from build123d import *

# Parameters (mm, degrees)
SKETCH1_R           = 10
SKETCH1_R_2         = 7.25
BOSS_EXTRUDE2_DEPTH = 10
SKETCH2_R           = 7.25
CUT_EXTRUDE1_DEPTH  = 10
CHAMFER5_SIZE       = 2.5
SKETCH5_W           = 6.2
SKETCH5_H           = 2
BOSS_EXTRUDE3_DEPTH = 8.5
SKETCH6_W           = 2.931408159
SKETCH6_H           = 6.9
BOSS_EXTRUDE4_DEPTH = 10
SKETCH7_W           = 8.5
SKETCH7_H           = 6.2
CUT_EXTRUDE2_DEPTH  = 1
SKETCH8_R           = 1.35
CUT_EXTRUDE3_DEPTH  = 20
BOSS_EXTRUDE5_START = -10
BOSS_EXTRUDE5_DEPTH = 10
SKETCH12_W          = 20
SKETCH12_H          = 10
SKETCH12_W_2        = 18
SKETCH12_H_2        = 8
BOSS_EXTRUDE7_DEPTH = 12
SKETCH13_W          = 10.931408159
SKETCH13_H          = 4.9
CUT_EXTRUDE4_DEPTH  = 9
SKETCH15_W          = 20
SKETCH15_H          = 10
SKETCH15_W_2        = 18
SKETCH15_H_2        = 8
CUT_EXTRUDE5_DEPTH  = 5


with BuildPart() as part:
    # Sketch1 → Boss-Extrude2 (new body)
    # profile 1 of 3: a face of its own
    with BuildSketch(Plane(origin=(0, 0, 0), x_dir=(1, 0, 0), z_dir=(0, 1, 0))):
        with Locations((-21.149759624, -29.701544489)):
            Circle(SKETCH1_R)
        with Locations((-21.149759624, -29.701544489)):
            Circle(SKETCH1_R_2, mode=Mode.SUBTRACT)
    # profile 2 of 3: a face of its own
    with BuildSketch(Plane(origin=(0, 0, 0), x_dir=(1, 0, 0), z_dir=(0, 1, 0))):
        with Locations((-21.149759624, -29.701544489)):
            Circle(SKETCH1_R_2)
    # profile 3 of 3: a face of its own
    with BuildSketch(Plane(origin=(0, 0, 0), x_dir=(1, 0, 0), z_dir=(0, 1, 0))):
        with BuildLine():
            Line((-1.149759624, -19.701544489), (-21.149759624, -19.701544489))
            ThreePointArc((-21.149759624, -19.701544489), (-14.078691812, -22.630476677), (-11.149759624, -29.701544489))
            ThreePointArc((-11.149759624, -29.701544489), (-14.078691797, -36.772612285), (-21.149759581, -39.701544489))
            Line((-21.149759581, -39.701544489), (-1.149759624, -39.701544489))
            Line((-1.149759624, -39.701544489), (-1.149759624, -32.801544489))
            Line((-1.149759624, -32.801544489), (-6.718351465, -32.801544489))
            Line((-6.718351465, -32.801544489), (-6.718351465, -26.601544489))
            Line((-6.718351465, -26.601544489), (-1.149759624, -26.601544489))
            Line((-1.149759624, -26.601544489), (-1.149759624, -19.701544489))
        make_face()
    extrude(amount=BOSS_EXTRUDE2_DEPTH)

    # Sketch2 → Cut-Extrude1 (cut)
    with BuildSketch(Plane(origin=(0, 10, 0), x_dir=(1, 0, 0), z_dir=(0, 1, 0))):
        with Locations(Location((-21.149759624, -29.701544489, 0), (0, 0, 270))):
            Circle(SKETCH2_R)
    extrude(amount=-CUT_EXTRUDE1_DEPTH, mode=Mode.SUBTRACT)

    # Chamfer5
    chamfer5_edges = [part.edges().sort_by_distance(p)[0] for p in [
        (-21.149759624, 0, 22.451544489),
        (-21.149759624, 10, 22.451544489),
    ]]
    chamfer(chamfer5_edges, length=CHAMFER5_SIZE)

    # Sketch5 → Boss-Extrude3 (add)
    with BuildSketch(Plane(origin=(-6.718351465, 0, 0), x_dir=(0, 0, -1), z_dir=(1, 0, 0))):
        with Locations((-29.701544489, 9)):
            Rectangle(SKETCH5_W, SKETCH5_H)
    extrude(amount=BOSS_EXTRUDE3_DEPTH)

    # Sketch6 → Boss-Extrude4 (add)
    with BuildSketch(Plane(origin=(0, 10, 0), x_dir=(1, 0, 0), z_dir=(0, 1, 0))):
        with Locations((0.315944456, -23.151544489)):
            Rectangle(SKETCH6_W, SKETCH6_H)
        with Locations((0.315944456, -36.251544489)):
            Rectangle(SKETCH6_W, SKETCH6_H)
    extrude(amount=-BOSS_EXTRUDE4_DEPTH)

    # Sketch7 → Cut-Extrude2 (cut)
    with BuildSketch(Plane.XZ.offset(-8)):
        with Locations((-2.468351465, 29.701544489)):
            Rectangle(SKETCH7_W, SKETCH7_H)
    extrude(amount=-CUT_EXTRUDE2_DEPTH, mode=Mode.SUBTRACT)

    # Sketch8 → Cut-Extrude3 (cut)
    with BuildSketch(Plane.XY.offset(39.701544489)):
        with Locations((-2.868351465, 5)):
            Circle(SKETCH8_R)
    extrude(amount=-CUT_EXTRUDE3_DEPTH, mode=Mode.SUBTRACT)

    # Sketch10 → Boss-Extrude5 (add)
    with BuildSketch(Plane(origin=(0, 10, 0), x_dir=(1, 0, 0), z_dir=(0, 1, 0)).offset(BOSS_EXTRUDE5_START)):
        with BuildLine():
            ThreePointArc((-31.149759624, -29.701544489), (-28.220827436, -22.630476677), (-21.149759624, -19.701544489))
            Line((-21.149759624, -19.701544489), (-31.149759624, -19.701544489))
            Line((-31.149759624, -19.701544489), (-31.149759624, -29.701544489))
        make_face()
        with BuildLine():
            ThreePointArc((-21.149759624, -39.701544489), (-28.220827436, -36.772612301), (-31.149759624, -29.701544489))
            Line((-31.149759624, -29.701544489), (-31.149759624, -39.701544489))
            Line((-31.149759624, -39.701544489), (-21.149759624, -39.701544489))
        make_face()
    extrude(amount=BOSS_EXTRUDE5_DEPTH)

    # Sketch12 → Boss-Extrude7 (add)
    with BuildSketch(Plane.ZY.offset(31.149759624)):
        with Locations((29.701544489, 5)):
            Rectangle(SKETCH12_W, SKETCH12_H)
        with Locations((29.701544489, 5)):
            Rectangle(SKETCH12_W_2, SKETCH12_H_2, mode=Mode.SUBTRACT)
    extrude(amount=BOSS_EXTRUDE7_DEPTH)

    # Sketch13 → Cut-Extrude4 (cut)
    with BuildSketch(Plane.XZ):
        with Locations((-4.684055545, 23.151544489)):
            Rectangle(SKETCH13_W, SKETCH13_H)
        Polygon((-13.850581564, 20.701544489), (-10.149759624, 25.601544489), (-10.149759624, 20.701544489), align=None)
        with Locations((-4.684055545, 36.251544489)):
            Rectangle(SKETCH13_W, SKETCH13_H)
        Polygon((-13.850581564, 38.701544489), (-10.149759624, 38.701544489), (-10.149759624, 33.801544489), align=None)
    extrude(amount=-CUT_EXTRUDE4_DEPTH, mode=Mode.SUBTRACT)

    # Sketch15 → Cut-Extrude5 (cut)
    with BuildSketch(Plane.ZY.offset(43.149759624)):
        with Locations((29.701544489, 5)):
            Rectangle(SKETCH15_W, SKETCH15_H)
        with Locations((29.701544489, 5)):
            Rectangle(SKETCH15_W_2, SKETCH15_H_2, mode=Mode.SUBTRACT)
    extrude(amount=-CUT_EXTRUDE5_DEPTH, mode=Mode.SUBTRACT)


solid = part.part
Check sheet for the modelled part. Datum: model origin and axes. Units: mm. A direction names the side the tool comes from. Give positions to 0.01 mm unless a question says otherwise; leave off trailing zeros. Loops run counter-clockwise (first coordinate to the right, second up) from the corner with the lowest first, then second, coordinate; pieces in that order, holes last. Notation, with made-up numbers: M -13.5,45 L -9.5,45 A16 cw -9.5,51 Z; hole C 0,42 d6. An arc over 180 degrees is marked long. Return JSON: item names as keys, results as strings. Group by question number.
1. Tool access check on faces 4 (the flat face through (-7, 4, 20.702)), 5 (the flat face through (-35, 5, 20.702)), 6 (the flat face through (-6.718, 4, 30)). Record the directions out of +Z, -Z, +X, -X, +Y, -Y that give a thin tool (end or side, any length) a straight path to the whole face; none if there is none.
2. Mould release check, pull along Z, two halves, no side actions. Record for faces 1 (the flat face through (-1, 4, 32.802)), 2 (the flat face through (-18, 5, 19.702)), 3 (the flat face through (1.782, 9.5, 29.8)): released by +Z, released by -Z, zero draft, split by the parting line, or undercut.
3. Go/stop test with flat-tipped pins: pin 1 (1.5 mm diameter, centred on x = -8, z = 35.5, fed in from -Y); pin 2 (1.5 mm diameter, centred on y = 7.5, z = 25.5, fed in from -X); pin 3 (2 mm diameter, centred on x = -2.87, y = 5, fed in from -Z). Record where each tip stops, or that it passes through.
4. Cross-section at B-B on x = -3. State how many separate pieces and enclosed holes the cut face has, plus the area to 3 significant figures.
5. Cross-section at A-A on x = -8. Record the boundary of the cut face in (y, z), plus the area to 3 significant figures.
6. Thickness scan on L1, parallel to Z at x = -9, y = 2.25; L2, parallel to Z at x = -5.5, y = 2.25; L3, parallel to Z at x = -33, y = 5. Record the ranges inside material, lowest first.
Return value:
{
 "1": {"face 4": "-Y", "face 5": "-X", "face 6": "+X, -Y"},
 "2": {"face 1": "undercut", "face 2": "released by -Z", "face 3": "zero draft"},
 "3": {"pin 1": "y = 9", "pin 2": "x = -31.15", "pin 3": "through"},
 "4": {"separate pieces": "5", "enclosed holes": "0", "area": "45.3 mm^2"},
 "5": {"outline": "M 0,19.7 L 10,19.7 L 10,39.7 L 0,39.7 L 0,38.7 L 9,38.7 L 9,33.8 L 0,33.8 L 0,25.6 L 9,25.6 L 9,20.7 L 0,20.7 Z", "area": "112 mm^2"},
 "6": {"L1": "19.7 to 20.7, 25.6 to 33.8, 38.7 to 39.7", "L2": "19.7 to 20.7, 25.6 to 26.6, 32.8 to 33.8, 38.7 to 39.7", "L3": "19.7 to 20.7, 38.7 to 39.7"}
}
